Autodesk Inventor part; units mm, degrees
ref_plane "Work Plane1" through (0, 0, -15) normal (0, 0, 1) x (1, 0, 0)
ref_plane "YZ Plane" through (0, 0, 0) normal (1, 0, 0) x (0, 1, 0)
ref_plane "XZ Plane" through (0, 0, 0) normal (0, 1, 0) x (-1, 0, 0)
sketch "Sketch1" plane through (0, 0, 0) normal (0, 0, 1) x (1, 0, 0)
  line L0 (0, 0) -> (25, 0)
  line L1 (25, 0) -> (25, 40)
  line L2 (25, 40) -> (0, 40)
  line L3 (0, 40) -> (0, 0)
  dimension "d1" = 25
  dimension "d2" = 40
  dimension "d3" = 25
extrude "Extrusion1" add sketch "Sketch1" against normal blind 30
sketch "Sketch2" plane through (25, 0, 0) normal (1, 0, 0) x (0, 0, -1)
  line L0 (0, 0) -> (30, 0)
  circle A0 centre (15, 6.56) radius 2.46
extrude "Extrusion2" cut sketch "Sketch2" against normal blind 30
sketch "Sketch3" plane through (0, 0, 0) normal (-1, 0, 0) x (0, 0, 1)
  line L0 (0, 0) -> (-30, 0)
  line L1 (-25.05, 0) -> (-4.95, 0)
  line L2 (-4.95, 0) -> (-4.95, 33.12)
  line L3 (-4.95, 33.12) -> (-25.05, 33.12)
  line L4 (-25.05, 33.12) -> (-25.05, 0)
  dimension "d11" = 20.1
extrude "Extrusion3" cut sketch "Sketch3" against normal blind 20
sketch "Sketch4" plane through (0, 0, 0) normal (0, -1, 0) x (1, 0, 0)
  line L0 (20, -4.95) -> (20, -25.05)
  line L1 (20, -15) -> (25, -15)
  line L2 (25, 0) -> (25, -30)
  line L3 (20, -8.025) -> (25, -8.025)
  line L4 (25, -8.025) -> (25, -21.975)
  line L5 (25, -21.975) -> (20, -21.975)
  line L6 (20, -21.975) -> (20, -8.025)
  line L7 (20, -8.025) -> (25, -21.975) construction
  line L8 (25, -8.025) -> (20, -21.975) construction
  line L9 (25, -12.54) -> (25, -17.46)
  point P0 (0, 0)
  point P1 (22.5, -15)
  dimension "d14" = 13.95
extrude "Extrusion4" add sketch "Sketch4" along normal blind 15
sketch "Sketch5" plane through (20, 0, 0) normal (-1, 0, 0) x (0, 0, 1)
  circle A0 centre (-15, 6.56) radius 2.46
  circle A1 centre (-15, 6.56) radius 4.7025
  circle A2 centre (-15, 6.56) radius 2.46
  circle A3 centre (-15, 6.56) radius 2.46
  point P0 (0, 0)
  dimension "d17" = 9.405
extrude "Extrusion5" cut sketch "Sketch5" against normal blind 2.1
sketch "Sketch6" plane through (25, 0, 0) normal (1, 0, 0) x (0, 0, -1)
  circle A0 centre (15, 6.56) radius 4.7025
  line L0 (15, 6.56) -> (15, 23.56)
  circle A1 centre (15, 23.56) radius 2.46
  point P0 (0, 0)
  dimension "d20" = 17
  dimension "d21" = 4.92
extrude "Extrusion6" cut sketch "Sketch6" against normal blind 10 contours A1
sketch "Sketch7" plane through (20, 0, 0) normal (-1, 0, 0) x (0, 0, 1)
  circle A0 centre (-15, 23.56) radius 2.46
  circle A1 centre (-15, 23.56) radius 4.7025
  point P0 (0, 0)
  dimension "d24" = 9.405
extrude "Extrusion7" cut sketch "Sketch7" against normal blind 2.1
sketch "Sketch9" plane through (25, 0, 0) normal (1, 0, 0) x (0, 0, -1)
  circle A0 centre (15, 6.56) radius 2.46
  circle A1 centre (15, 6.56) radius 2.46
  circle A2 centre (15, 23.56) radius 2.46
  circle A3 centre (15, 23.56) radius 2.46
  line L0 (30, 40) -> (30, 0)
  line L1 (30, 0) -> (30, 40)
  line L2 (30, 40) -> (0, 40)
  line L3 (0, 40) -> (0, 0)
  line L4 (0, 0) -> (8.025, 0)
  line L5 (21.975, 0) -> (21.975, -15)
  line L6 (21.975, -15) -> (8.025, -15)
  line L7 (8.025, -15) -> (8.025, 0)
  line L8 (0, 0) -> (8.025, 0)
  line L9 (21.975, 0) -> (30, 0)
extrude "Extrusion8" add sketch "Sketch9" along normal blind 5
sketch "Sketch10" plane through (0, 40, 0) normal (0, 1, 0) x (1, 0, 0)
  line L0 (0, 30) -> (30, 30)
  line L1 (30, 0) -> (0, 0)
  line L2 (0, 30) -> (30, 30)
  line L3 (30, 30) -> (30, 0)
  line L4 (30, 0) -> (0, 0)
  line L5 (0, 0) -> (0, 30)
extrude "Extrusion9" add sketch "Sketch10" along normal blind 30
sketch "Sketch12" plane through (30, 0, 0) normal (1, 0, 0) x (0, 0, -1)
  circle A0 centre (15, 6.56) radius 2.46
  line L0 (15, 6.56) -> (15, 15.06)
  circle A1 centre (15, 15.06) radius 2.525
  point P0 (0, 0)
  dimension "d31" = 8.5
  dimension "d33" = 5.05
extrude "Extrusion10" cut sketch "Sketch12" against normal blind 30 contours A1
sketch "Sketch14" plane through (0, 0, 0) normal (0, 0, 1) x (1, 0, 0)
  line L0 (30, 70) -> (0, 70)
  line L1 (0, 100) -> (-8, 100)
  line L2 (30, 0) -> (30, 70)
  line L3 (30, 118) -> (30, 70)
  line L4 (30, 105) -> (30, 100)
  line L5 (0, 70) -> (30, 70)
  line L6 (0, 70) -> (0, 100)
  line L7 (30, 122.5) -> (30, 118)
  line L8 (-2, 150) -> (-8, 152)
  line L9 (-2, 102) -> (-8, 100)
  line L10 (-2, 102) -> (4, 126)
  line L11 (4, 126) -> (-2, 150)
  line L12 (-8, 152) -> (15, 152)
  line L13 (30, 137) -> (15, 152)
  line L14 (30, 122.5) -> (30, 137)
  point P0 (0, 0)
  dimension "d47" = 30
extrude "Extrusion12" add sketch "Sketch14" against normal blind 30
sketch "Sketch15" plane through (0, 0, -25.05) normal (-1, 0, 0) x (0, 0, 1)
  line L0 (0, 33.12) -> (20.1, 33.12)
  line L1 (20.1, 33.12) -> (20.1, 0)
  line L2 (0, 33.12) -> (20.1, 33.12)
  line L3 (20.1, 33.12) -> (20.1, 31.1)
  line L4 (20.1, 31.1) -> (0, 31.1)
  line L5 (0, 31.1) -> (0, 33.12)
  point P0 (25.05, 0)
  dimension "d57" = 2.02
extrude "Extrusion13" add sketch "Sketch15" against normal blind 20
sketch "Sketch25" plane through (0, 0, 0) normal (0, 0, 1) x (1, 0, 0)
  point P0 (0, 0)
sketch "Sketch26" plane through (0, 0, 0) normal (0, 0, 1) x (1, 0, 0)
  line L0 (-8, 100) -> (0, 100)
  line L1 (0, 100) -> (-8, 100)
  line L2 (-8, 100) -> (-2, 102)
  line L3 (-8, 100) -> (-2, 102)
  line L4 (-2, 102) -> (4, 126)
  line L5 (-2, 102) -> (4, 126)
  line L6 (4, 126) -> (-2, 150)
  line L7 (4, 126) -> (-2, 150)
  line L8 (-8, 152) -> (-2, 150)
  line L9 (-2, 150) -> (-8, 152)
  line L10 (15, 152) -> (-8, 152)
  line L11 (-8, 152) -> (15, 152)
  line L12 (30, 137) -> (15, 152)
  line L13 (15, 152) -> (30, 137)
  line L14 (30, 137) -> (30, 92)
  line L15 (30, 0) -> (30, 137)
  line L16 (30, 92) -> (0, 92)
  line L17 (0, 0) -> (0, 100)
  line L18 (0, 100) -> (0, 92)
  dimension "d93" = 45
extrude "Extrusion14" add sketch "Sketch26" along normal blind 15
ref_plane "Work Plane1" through (0, 0, -15) normal (0, 0, 1) x (1, 0, 0)
mirror "Mirror1" about plane through (0, 0, -15) normal (0, 0, 1) of "Extrusion14"
properties part number "48mm_x_60mm"
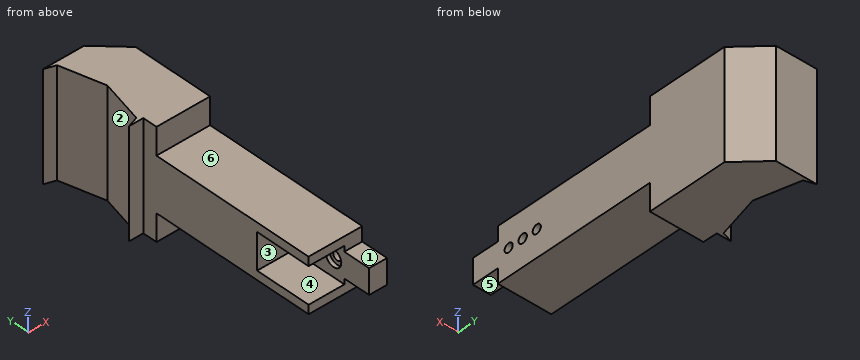
Could you check a few things on this model? Use its own coordinates, in mm. Face numbers are marked on the shaded views. A direction names the side the tool comes from. Round coordinates to 2 decimals unless told otherwise and drop trailing zeros. Loops run counter-clockwise (first coordinate to the right, second up) from the corner with the lowest first, then second, coordinate; pieces in that order, holes last.
Q1. I want a section at D-D (x = 27). Write out the boundary of the cut face in (y, z) (3 decimals).
Q2. I want a section at B-B (y = 23.56). Write out the boundary of the cut face in (x, z), and give its area (3 significant figures).
Q3. On a 3-axis mill with a long thin cutter (end or side, diameter ignored), from which of +Z, -Z, +X, -X, +Y, -Y can I reach the whole of each face in a straight line? I mean the marked faces 4, 5 and 6. Say none if no direction works.
Q4. I want a section at C-C (z = -15). Give the number of separate pieces and of enclosed holes in the cut face, and give its area (3 significant figures).
Q5. For P1, Ø9, axis at x = 12, y = 35, coming from the +Z side; P2, Ø3, axis at y = 9, z = -15, coming from the -X side; P3, Ø5, axis at y = 86, z = -3, coming from the -X side, each with a flat end and sliding along its axis, tell me the tip position at first contact or that it passes through.
Q6. Thinking about a two-plate mould opening in Z: for the marked faces 1, 2 and 3, which applies, pulls with the +Z half, pulls with the -Z half, needs draft (parallel to the pull), parting line crosses it, or undercut?
Q7. I want a section at A-A (x = -5). Write out the boundary of the cut face in (y, z).
Q8. Please list where these lines run through material, in increasing order: L1, parallel to Y at x = 25.5, z = -15 (3 decimals); L2, parallel to Z at x = 13, y = 22.5; L3, parallel to Y at x = 27, z = -15 (3 decimals).
Answer below:
1. outline: (-15, -21.975) - (0, -21.975) - (0, -30) - (92, -30) - (92, -45) - (140, -45) - (140, 15) - (92, 15) - (92, 0) - (0, 0) - (0, -8.025) - (-15, -8.025) - close; hole circle Ø4.92 at (6.56, -15); hole circle Ø5.05 at (15.06, -15); hole circle Ø4.92 at (23.56, -15)
2. outline: (0, -30) - (30, -30) - (30, -17.46) - (22.1, -17.46) - (22.1, -19.7) - (20, -19.7) - (20, -25.05) - (0, -25.05) - close; (0, -4.95) - (20, -4.95) - (20, -10.3) - (22.1, -10.3) - (22.1, -12.54) - (30, -12.54) - (30, 0) - (0, 0) - close
2. area: 439 mm2
3. face 4: -X, -Y
3. face 5: -Z, +X, -X, -Y
3. face 6: +Z, +X, -X, -Y
4. separate pieces: 4
4. enclosed holes: 0
4. area: 3,780 mm2
5. P1: stops at z = 0
5. P2: stops at x = 22.1
5. P3: stops at x = 0
6. face 1: pulls with the +Z half
6. face 2: needs draft
6. face 3: undercut
7. outline: (100, -45) - (101, -45) - (101, 15) - (100, 15) - close; (151, -45) - (152, -45) - (152, 15) - (151, 15) - close
8. L1: y = -15 to 4.1, 9.02 to 12.535, 17.585 to 21.1, 26.02 to 141.5
8. L2: z = -30 to -25.05, -4.95 to 0
8. L3: y = -15 to 4.1, 9.02 to 12.535, 17.585 to 21.1, 26.02 to 140
